```python
from build123d import *

# Parameters (mm, degrees)
F1_DEPTH = 25.4
F3_DEPTH = 7.62
F4_W     = 5.08
F4_H     = 17.78
F5_DEPTH = 12.7


with BuildPart() as f1:
    # F0 (on Top) → F1 (new body)
    with BuildSketch(Plane.XY):
        with BuildLine():
            ThreePointArc((0, 8.89), (8.89, 0), (0, -8.89))
            Line((0, -8.89), (0, -13.97))
            ThreePointArc((0, -13.97), (13.97, 0), (0, 13.97))
            Line((0, 13.97), (0, 8.89))
        make_face()
    extrude(amount=F1_DEPTH)

    # F2 (on face) → F3 (join)
    with BuildSketch(Plane(origin=(0, 0, 0), x_dir=(1, 0, 0), z_dir=(0, 0, -1))):
        with BuildLine():
            Line((100.33, 8.89), (10.7763073453, 8.89))
            ThreePointArc((10.7763073453, 8.89), (13.97, 0), (10.7763073453, -8.89))
            Line((10.7763073453, -8.89), (100.33, -8.89))
            Line((100.33, -8.89), (100.33, 8.89))
        make_face()
    extrude(amount=-F3_DEPTH)

    # F4 (on face) → F5 (join)
    with BuildSketch(Plane.XY.offset(7.62)):
        with Locations((97.79, 0)):
            Rectangle(F4_W, F4_H)
    extrude(amount=F5_DEPTH)


solid = f1.part
```
Work out the finished part from the listing and answer in its coordinate system (mm). A direction names the side the tool comes from. Round coordinates to 2 decimals unless told otherwise and drop trailing zeros. Write each loop counter-clockwise with the first axis right and the second up, starting at its lowest first coordinate (ties: lowest second). Pieces come first, ordered by that corner, then holes.
1) Determine the mould class of faces 1 (the face through (59, 8.89, 4)), 2 (the face through (8.888, 0.195, 12.522)), 3 (the face through (59, -8.89, 4)), 4 (the face through (0, 11, 13)) for opening direction Y: pulls with the +Y half, pulls with the -Y half, needs draft (parallel to the pull), parting line crosses it, or undercut.
2) Which of the six approach directions +Z, -Z, +X, -X, +Y, -Y give full straight-line access (tool end or side, diameter ignored) to faces 5 (the face through (10, 0, 25.4)), 6 (the face through (13.967, -0.307, 15.344)), 7 (the face through (98, 0, 20.32)), 8 (the face through (95.25, 0, 14))?
3) Consider probe 1 along Z at (x, y) = (35.5, -3.5); probe 2 along Y at (x, z) = (28.5, 6.75); probe 3 along X at (y, z) = (-3, 11.25). Determine where each line is inside the solid, lowest interval first.
4) A cutting plane is placed at D-D on x = 17.5. Determine the outline of the cut face in (y, z), and give its area (3 significant figures).
5) A cutting plane is placed at A-A on z = 18. Determine the outline of the cut face in (x, y), and give its area (3 significant figures).
6) Flat-ended cylindrical pins translate along their axes: P1, Ø4, axis at x = 77, z = 3, coming from the -Y side; P2, Ø3, axis at x = 14, z = 21, coming from the +Y side; P3, Ø14, axis at y = 2.5, z = 12, coming from the -X side; P4, Ø4, axis at x = 99, y = -3, coming from the +Z side. Find the tip coordinate at first contact, or state that the pin passes through.
7) A cutting plane is placed at C-C on z = 3. Determine the outline of the cut face in (x, y), and give its area (3 significant figures).
8) A cutting plane is placed at B-B on y = -2.75. Determine the outline of the cut face in (x, z).
Entries:
1. face 1: pulls with the +Y half
1. face 2: undercut
1. face 3: pulls with the -Y half
1. face 4: needs draft
2. face 5: +Z, +X, -X, +Y, -Y
2. face 6: +Z
2. face 7: +Z, +X, +Y, -Y
2. face 8: +Z, +Y, -Y
3. probe 1: z = 0 to 7.62
3. probe 2: y = -8.89 to 8.89
3. probe 3: x = 8.37 to 13.64, 95.25 to 100.33
4. outline: (-8.89, 0) - (8.89, 0) - (8.89, 7.62) - (-8.89, 7.62) - close
4. area: 135 mm2
5. outline: (0, -13.97) arc R13.97 ccw to (0, 13.97) - (0, 8.89) arc R8.89 cw to (0, -8.89) - close; (95.25, -8.89) - (100.33, -8.89) - (100.33, 8.89) - (95.25, 8.89) - close
5. area: 273 mm2
6. P1: stops at y = -8.89
6. P2: stops at y = 6.24
6. P3: stops at x = 0
6. P4: stops at z = 20.32
7. outline: (0, -13.97) arc R13.97 ccw to (10.78, -8.89) - (100.33, -8.89) - (100.33, 8.89) - (10.78, 8.89) arc R13.97 ccw to (0, 13.97) - (0, 8.89) arc R8.89 cw to (0, -8.89) - close
7. area: 1,740 mm2
8. outline: (8.45, 0) - (100.33, 0) - (100.33, 20.32) - (95.25, 20.32) - (95.25, 7.62) - (13.7, 7.62) - (13.7, 25.4) - (8.45, 25.4) - close
